Autodesk Inventor part; units mm, degrees
ref_plane "YZ Plane" through (0, 0, 0) normal (1, 0, 0) x (0, 1, 0)
ref_plane "XY Plane" through (0, 0, 0) normal (0, 0, 1) x (1, 0, 0)
ref_plane "作業平面2" through (0, 6.5, 0) normal (0, 1, 0) x (-1, 0, 0)
sketch "スケッチ3" plane through (0, 6.5, 0) normal (0, 1, 0) x (-1, 0, 0)
  line L0 (4.725, -4.725) -> (-4.725, -4.725)
  line L1 (-4.725, -4.725) -> (-4.725, 4.725)
  line L2 (-4.725, 4.725) -> (4.725, 4.725)
  line L3 (4.725, 4.725) -> (4.725, -4.725)
  line L4 (4.725, -4.725) -> (-4.725, 4.725) construction
  line L5 (-4.725, -4.725) -> (4.725, 4.725) construction
  line L6 (5.8, -5.8) -> (-5.8, -5.8)
  line L7 (-5.8, -5.8) -> (-5.8, 5.8)
  line L8 (-5.8, 5.8) -> (5.8, 5.8)
  line L9 (5.8, 5.8) -> (5.8, -5.8)
  line L10 (5.8, -5.8) -> (-5.8, 5.8) construction
  line L11 (-5.8, -5.8) -> (5.8, 5.8) construction
  point P0 (0, 0)
  point P1 (0, 0)
  dimension "d19" = 9.45
  dimension "d20" = 9.45
  dimension "d21" = 11.6
  dimension "d22" = 11.6
sketch "スケッチ1" plane through (0, 0, 0) normal (0, 1, 0) x (-1, 0, 0)
  line L0 (6.5, -6.5) -> (-6.5, 6.5) construction
  line L1 (-6.5, -6.5) -> (6.5, 6.5) construction
  line L2 (1.0609, 3.9595) -> (3.9595, 1.0609)
  line L3 (3.9595, 1.0609) -> (2.8986, -2.8986)
  line L4 (2.8986, -2.8986) -> (-1.0609, -3.9595)
  line L5 (-1.0609, -3.9595) -> (-3.9595, -1.0609)
  line L6 (-3.9595, -1.0609) -> (-2.8986, 2.8986)
  line L7 (-2.8986, 2.8986) -> (1.0609, 3.9595)
  line L8 (-6.5, -6.5) -> (6.5, -6.5)
  line L9 (6.5, -6.5) -> (6.5, 6.5)
  line L10 (6.5, 6.5) -> (-6.5, 6.5)
  line L11 (-6.5, 6.5) -> (-6.5, -6.5)
  line L12 (-6.5, -6.5) -> (6.5, 6.5) construction
  line L13 (6.5, -6.5) -> (-6.5, 6.5) construction
  circle A0 centre (0, 0) radius 2.4
  dimension "d33" = 7.1
  dimension "d34" = 13
  dimension "d35" = 13
  dimension "d36" = 4.8
extrude "押し出し8" add sketch "スケッチ1" along normal blind 6.5 contours L2 L3 L4 L5 L6 L7 | L11 L10 L9 L8 | A0
extrude "押し出し9" cut sketch "スケッチ3" against normal blind 2
extrude "押し出し10" cut sketch "スケッチ1" along normal blind 3.5 contours L2 L3 L4 L5 L6 L7
extrude "押し出し11" cut sketch "スケッチ1" along normal blind 6.5 contours A0
fillet "フィレット2" radius 1 4 edges at (-6.5, 0, 0) (0, 0, 6.5) (0, 0, -6.5) (6.5, 0, 0)
fillet "フィレット3" radius 0.3 1 edges at (2.4, 6.5, 0)
fillet "フィレット4" radius 0.3 1 edges at (2.4, 3.5, 0)
equation "\"d20\" = d19"
equation "\"d22\" = d21"
properties part number "pin_joint_ver1"
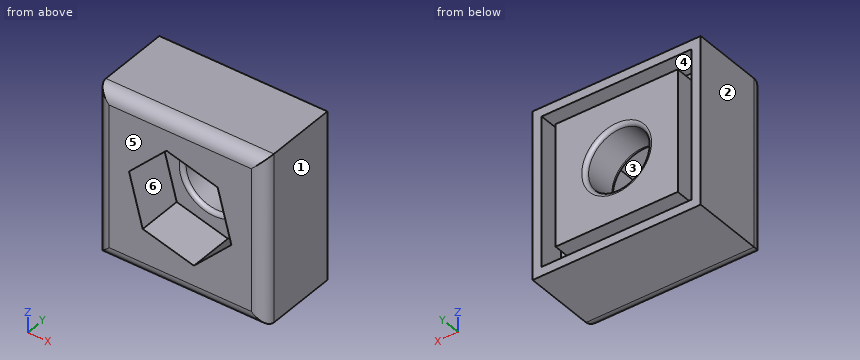
Could you check a few things on this model? Use its own coordinates, in mm. Face numbers are marked on the shaded views. A direction names the side the tool comes from. Round coordinates to 2 decimals unless told otherwise and drop trailing zeros. Write each loop counter-clockwise with the first axis right and the second up, starting at its lowest first coordinate (ties: lowest second). Pieces come first, ordered by that corner, then holes. Notation, with made-up numbers: (69, 13.5) - (82, 13.5) arc R25 ccw to (82, 38.5) - close; hole circle Ø9 at (-22.75, -19). An arc over 180 degrees is marked (long way). Put each result on its own line as item: value. Start each with the question number.
(1) Will this pin go through, and if not, where does the flat tip stop? pin 1 (6 mm diameter, centred on x = 0, z = 0, fed in from +Y).
(2) I need wall thicknesses on probe 1 along Z at (x, y) = (0, 5.65) (3 decimals); probe 2 along Z at (x, y) = (-3.5, 5.25) (3 decimals); probe 3 along Z at (x, y) = (5, 4.75). Which ranges of each line are inside material? Lowest first, please.
(3) I want a section at A-A, the plane y = 2. Please give me the cut outline in (x, z).
(4) Thinking about a two-plate mould opening in X: for the marked faces 1, 2 and 3, which applies, released by +X, released by -X, zero draft, split by the parting line, or undercut?
(5) For the marked faces 4, 5 and 6, which set-ups out of +Z, -Z, +X, -X, +Y, -Y let a thin tool reach every point of the face, with its end or its side?
(6) I want a section at B-B, the plane x = 0. Please give me the cut outline in (y, z) (3 decimals).
(7) I want a section at C-C, the plane z = 0. Please give me the cut outline in (x, y) (3 decimals).
Here are the results:
1. pin 1: stops at y = 6.5
2. probe 1: z = -6.5 to -5.8, -4.725 to -2.4, 2.4 to 4.725, 5.8 to 6.5
2. probe 2: z = -6.5 to -5.8, -4.725 to 4.725, 5.8 to 6.5
2. probe 3: z = -6.5 to -5.8, 5.8 to 6.5
3. outline: (-6.5, -6.5) - (6.5, -6.5) - (6.5, 6.5) - (-6.5, 6.5) - close; hole (-3.96, 1.06) - (-2.9, -2.9) - (1.06, -3.96) - (3.96, -1.06) - (2.9, 2.9) - (-1.06, 3.96) - close
4. face 1: released by +X
4. face 2: released by -X
4. face 3: undercut
5. face 4: +Y
5. face 5: +Z, -Z, +X, -X, -Y
5. face 6: -Y
6. outline: (0, -5.5) arc R1 ccw to (1, -6.5) - (6.5, -6.5) - (6.5, -5.8) - (4.5, -5.8) - (4.5, -4.725) - (6.5, -4.725) - (6.5, -2.7) arc R0.3 ccw to (6.2, -2.4) - (3.8, -2.4) arc R0.3 ccw to (3.5, -2.7) - (3.5, -3.675) - (0, -3.675) - close; (0, 3.675) - (3.5, 3.675) - (3.5, 2.7) arc R0.3 ccw to (3.8, 2.4) - (6.2, 2.4) arc R0.3 ccw to (6.5, 2.7) - (6.5, 4.725) - (4.5, 4.725) - (4.5, 5.8) - (6.5, 5.8) - (6.5, 6.5) - (1, 6.5) arc R1 ccw to (0, 5.5) - close
7. outline: (-6.5, 1) arc R1 ccw to (-5.5, 0) - (-3.675, 0) - (-3.675, 3.5) - (-2.7, 3.5) arc R0.3 ccw to (-2.4, 3.8) - (-2.4, 6.2) arc R0.3 ccw to (-2.7, 6.5) - (-4.725, 6.5) - (-4.725, 4.5) - (-5.8, 4.5) - (-5.8, 6.5) - (-6.5, 6.5) - close; (2.4, 3.8) arc R0.3 ccw to (2.7, 3.5) - (3.675, 3.5) - (3.675, 0) - (5.5, 0) arc R1 ccw to (6.5, 1) - (6.5, 6.5) - (5.8, 6.5) - (5.8, 4.5) - (4.725, 4.5) - (4.725, 6.5) - (2.7, 6.5) arc R0.3 ccw to (2.4, 6.2) - close
